Design review of the part built by this model. Coordinates are the model's own, in mm. A direction names the side the tool comes from. Give positions to 0.01 mm unless a question says otherwise; leave off trailing zeros. Write each loop counter-clockwise with the first axis right and the second up, starting at its lowest first coordinate (ties: lowest second). Pieces come first, ordered by that corner, then holes. Notation, with made-up numbers: (79.25, 76.25) -> (108.25, 76.25) arc R26 cw to (108.25, 108.25) -> close; hole circle Ø4 at (25.5, 62). An arc over 180 degrees is marked (long way). Answer as a JSON object with one key per item and string values.
```python
from build123d import *

# Parameters (mm, degrees)
F1_DEPTH = 150
F2_DEPTH = 25
F2_TAPER = -50
F3_R     = 36.2779782861
F4_DEPTH = 30


with BuildPart() as f1:
    # F0 (on Front) → F1 (new body)
    with BuildSketch(Plane.XZ):
        Polygon((-16.5601376103, -17.1414369862), (28.5954256631, -16.5359374457), (5.4932660423, 22.267177701), align=None)
    extrude(amount=F1_DEPTH)

    # F1_face (on face) → F2 (join)
    with BuildSketch(Plane(origin=(5.842851365, 0, -3.8033989103), x_dir=(1, 0, 0), z_dir=(0, 1, 0))):
        Polygon((-22.4029889753, 13.3380380759), (-0.3495853227, -26.0705766113), (22.752574298, 12.7325385354), align=None)
    extrude(amount=F2_DEPTH, taper=F2_TAPER)

    # F3 (on face) → F4 (join)
    with BuildSketch(Plane(origin=(0, 25, 0), x_dir=(-1, 0, 0), z_dir=(0, 1, 0))):
        with Locations((-4.6302080154, 0)):
            Circle(F3_R)
    extrude(amount=F4_DEPTH)


solid = f1.part
```
(1) We need section A-A, the plane y = -107. State the section outline as (x, z) points, then the cut area to 3 significant figures.
Here are the results:
{"outline": "(-16.56, -17.14) -> (28.6, -16.54) -> (5.49, 22.27) -> close", "area": "883 mm²"}
(2) For line 1 along X through (y, z) = (1.5, -4); line 2 along X through (y, z) = (32.5, 2); line 3 along Y through (x, z) = (11, 57), list the stretches that pass through material, from the lowest coordinate up.
Here are the results:
{"line 1": "x = -11.25 to 23.21", "line 2": "x = -31.59 to 40.85", "line 3": "y = 18.88 to 25"}
(3) Clearance check with flat-ended pins moving along their axes: pin 1 (4 mm diameter, centred on x = 24.5, z = -0.5, fed in from -Y); pin 2 (3 mm diameter, centred on y = -76, z = 11, fed in from +X); pin 3 (6 mm diameter, centred on y = 11, z = 14.5, fed in from -X). State where each tip first meets the part, or that it passes through.
Here are the results:
{"pin 1": "stops at y = 2.25", "pin 2": "stops at x = 13.09", "pin 3": "stops at x = -18.3"}
(4) For faces 1 (the flat face through (6, -150, -2)), 2 (the flat face through (5, 55, 1)), 3 (the flat face through (-5.4, -74, 2.8)), 4 (the cylindrical face through (33.4, 39.8, -22.1)), 5 (the flat face through (17.21, -73.95, 2.59)), list the 3-axis set-ups (+Z, -Z, +X, -X, +Y, -Y) from which the entire face can be reached by the end or side of a thin tool; tool diameter is ignored.
Here are the results:
{"face 1": "+Z, -Z, +X, -X, -Y", "face 2": "+Z, -Z, +X, -X, +Y", "face 3": "+Z, -X, -Y", "face 4": "+Y", "face 5": "+Z, +X, -Y"}
